Read the model definition and answer for the solid it produces. Units are mm, in the model's axes. Give positions to 0.01 mm unless a question says otherwise; leave off trailing zeros. Write each loop counter-clockwise with the first axis right and the second up, starting at its lowest first coordinate (ties: lowest second). Pieces come first, ordered by that corner, then holes.
```python
from build123d import *

# Parameters (mm, degrees)
F0_R            = 50.8
F0_R_2          = 14.1605
F1_DEPTH        = 3.175
F2_R            = 2.3622
F3_DEPTH        = 3.176
F3_COPIES_COUNT = 6


# Not quite as in the source:
# - a pattern or mirror of a feature is missing from the dataset's text; its kind, count and spacing are read off the source's solid


with BuildPart() as f1:
    # F0 (on Top) → F1 (new body)
    with BuildSketch(Plane.XY):
        Circle(F0_R)
        Circle(F0_R_2, mode=Mode.SUBTRACT)
    extrude(amount=F1_DEPTH)

    # F2 (on face) → F3 (cut, through all)
    with BuildSketch(Plane.XY.offset(3.175)):
        with Locations((0, 23.8125)):
            Circle(F2_R)
    f3 = extrude(amount=-F3_DEPTH, mode=Mode.SUBTRACT)

    # F3_copies: F3 ×6 about axis
    f3_copies_axis = Axis((0, 0, 0), (0, 0, 1))
    for i in range(1, F3_COPIES_COUNT):
        add(f3.rotate(f3_copies_axis, i * 360 / F3_COPIES_COUNT), mode=Mode.SUBTRACT)


solid = f1.part
```
Item 1: Section A-A (y = 0) is taken. Write down the section's boundary in (x, z) (1 decimal).
Result set:
outline: (-50.8, 0) - (-14.2, 0) - (-14.2, 3.2) - (-50.8, 3.2) - close; (14.2, 0) - (50.8, 0) - (50.8, 3.2) - (14.2, 3.2) - close
Item 2: Section D-D (y = -25) is taken. Write down the section's boundary in (x, z) (3 decimals), and give its area (3 significant figures).
Result set:
outline: (-44.223, 0) - (-2.042, 0) - (-2.042, 3.175) - (-44.223, 3.175) - close; (2.042, 0) - (44.223, 0) - (44.223, 3.175) - (2.042, 3.175) - close
area: 268 mm2
Item 3: Find the intervals of material crossed by line 1 along Y through (x, z) = (0, 2.05); line 2 along Y through (x, z) = (-19, 1.7); line 3 along Y through (x, z) = (-22, 1.9), in increasing order.
Result set:
line 1: y = -50.8 to -26.17, -21.45 to -14.16, 14.16 to 21.45, 26.17 to 50.8
line 2: y = -47.11 to -13.62, -10.19 to 10.19, 13.62 to 47.11
line 3: y = -45.79 to -13.83, -9.99 to 9.99, 13.83 to 45.79
Item 4: Section B-B (x = 0) is taken. Write down the section's boundary in (y, z) (1 decimal), and give its area (3 significant figures).
Result set:
outline: (-50.8, 0) - (-26.2, 0) - (-26.2, 3.2) - (-50.8, 3.2) - close; (-21.5, 0) - (-14.2, 0) - (-14.2, 3.2) - (-21.5, 3.2) - close; (14.2, 0) - (21.5, 0) - (21.5, 3.2) - (14.2, 3.2) - close; (26.2, 0) - (50.8, 0) - (50.8, 3.2) - (26.2, 3.2) - close
area: 203 mm2
Item 5: Each of these flat-tipped pins is pushed along its axis until it touches: pin 1 Ø4.5 at (x, y) = (0, -23.81) entering from -Z; pin 2 Ø7.5 at (x, y) = (20.62, -11.91) entering from +Z (3 decimals). Where does it stop, or does it pass through?
Result set:
pin 1: passes through
pin 2: stops at z = 3.175
Item 6: Determine the mould class of faces 1 (the flat face through (11, -11, 3.175)), 2 (the cylindrical face through (-0.308, 26.155, 1.61)), 3 (the cylindrical face through (-22.875, 11.197, 1.61)), 4 (the cylindrical face through (-11.012, -49.592, 1.565)) for opening direction X: pulls with the +X half, pulls with the -X half, needs draft (parallel to the pull), parting line crosses it, or undercut.
Result set:
face 1: needs draft
face 2: undercut
face 3: undercut
face 4: parting line crosses it
Item 7: Section C-C (z = 1.05) is taken. Write down the section's boundary in (x, y).
Result set:
outline: circle Ø101.6 at (0, 0); hole circle Ø4.72 at (-20.62, -11.91); hole circle Ø4.72 at (-20.62, 11.91); hole circle Ø28.32 at (0, 0); hole circle Ø4.72 at (0, -23.81); hole circle Ø4.72 at (0, 23.81); hole circle Ø4.72 at (20.62, -11.91); hole circle Ø4.72 at (20.62, 11.91)
